The listing builds one solid part. Answer for the finished solid, in the listing's coordinates (mm). A direction names the side the tool comes from. Round coordinates to 2 decimals unless told otherwise and drop trailing zeros. Order: outer loops, then holes, each group sorted by start corner. A loop starts at its lowest first (then second) coordinate and runs counter-clockwise, first axis right, second up. Notation, with made-up numbers: (-5, 2.5) - (50, 2.5) arc R28 ccw to (50, 34.5) - close; hole circle Ø2 at (26.5, 81.25). An arc over 180 degrees is marked (long way). Write item = value, one per line.
from build123d import *

# Parameters (mm, degrees)
MODEL_W             = 85.14935
MODEL_H             = 104.19946
MODEL_W_2           = 77.14935
MODEL_H_2           = 96.19946
EXTRUDE_2_DEPTH     = 5
SKETCH_2_W          = 3.5
SKETCH_2_H          = 6
CUT_EXTRUDE_1_DEPTH = 2
SKETCH_4_W          = 91.14935
SKETCH_4_H          = 110.19946
SKETCH_4_W_2        = 85.14935
SKETCH_4_H_2        = 104.19946
EXTRUDE_5_DEPTH     = 20
FILLET_1_R          = 2
CHAMFER_1_SIZE      = 1
FILLET_2_R          = 1
CUT_EXTRUDE_2_DEPTH = 10


with BuildPart() as part:
    # Model → 凸台-拉伸2 (new body)
    with BuildSketch(Plane.XY):
        with Locations((38.194325, 47.88337)):
            Rectangle(MODEL_W, MODEL_H)
        with Locations((38.194325, 47.88337)):
            Rectangle(MODEL_W_2, MODEL_H_2, mode=Mode.SUBTRACT)
    extrude(amount=EXTRUDE_2_DEPTH)

    # 草图2 → 切除-拉伸1 (cut)
    with BuildSketch(Plane.XY.offset(5)):
        with Locations((-2.13035, 77.88337)):
            Rectangle(SKETCH_2_W, SKETCH_2_H)
        with Locations((78.519, 77.88337)):
            Rectangle(SKETCH_2_W, SKETCH_2_H)
        with Locations((-2.13035, 47.88337)):
            Rectangle(SKETCH_2_W, SKETCH_2_H)
        with Locations((78.519, 47.88337)):
            Rectangle(SKETCH_2_W, SKETCH_2_H)
        with Locations((-2.13035, 17.88337)):
            Rectangle(SKETCH_2_W, SKETCH_2_H)
        with Locations((78.519, 17.88337)):
            Rectangle(SKETCH_2_W, SKETCH_2_H)
    extrude(amount=-CUT_EXTRUDE_1_DEPTH, mode=Mode.SUBTRACT)

    # 草图4 → 凸台-拉伸5 (add)
    with BuildSketch(Plane(origin=(0, 0, 0), x_dir=(-1, 0, 0), z_dir=(0, 0, -1))):
        with Locations((-38.194325, 47.88337)):
            Rectangle(SKETCH_4_W, SKETCH_4_H)
        with Locations((-38.194325, 47.88337)):
            Rectangle(SKETCH_4_W_2, SKETCH_4_H_2, mode=Mode.SUBTRACT)
    extrude(amount=-EXTRUDE_5_DEPTH)

    # 圆角1
    fillet_1_edges = [part.edges().sort_by_distance(p)[0] for p in [
        (83.769, 102.9831, 10),
        (-7.38035, 102.9831, 10),
        (-7.38035, -7.21636, 10),
        (83.769, -7.21636, 10),
    ]]
    fillet(fillet_1_edges, radius=FILLET_1_R)

    # 倒角1
    chamfer_1_edges = [part.edges().sort_by_distance(p)[0] for p in [
        (-7.38035, 47.88337, 20),
        (38.194325, 102.9831, 20),
        (38.194325, -7.21636, 20),
        (83.769, 47.88337, 20),
        (-6.794563562, -6.630573562, 20),
        (83.183213562, -6.630573562, 20),
        (83.183213562, 102.397313562, 20),
        (-6.794563562, 102.397313562, 20),
    ]]
    chamfer(chamfer_1_edges, length=CHAMFER_1_SIZE)

    # 圆角2
    fillet_2_edges = [part.edges().sort_by_distance(p)[0] for p in [
        (-7.38035, 47.88337, 0),
        (38.194325, 102.9831, 0),
        (83.769, 47.88337, 0),
        (38.194325, -7.21636, 0),
        (-6.794563562, -6.630573562, 0),
        (83.183213562, -6.630573562, 0),
        (83.183213562, 102.397313562, 0),
        (-6.794563562, 102.397313562, 0),
    ]]
    fillet(fillet_2_edges, radius=FILLET_2_R)

    # 草图5 → 切除-拉伸2 (cut)
    with BuildSketch(Plane(origin=(76.38865, -7.21636, 20), x_dir=(-1, 0, 0), z_dir=(0, -1, 0))):
        with BuildLine():
            Line((33.694325, 13.169990539), (42.694325, 13.169990539))
            ThreePointArc((42.694325, 13.169990539), (45.094325, 10.769990539), (42.694325, 8.369990539))
            Line((42.694325, 8.369990539), (33.694325, 8.369990539))
            ThreePointArc((33.694325, 8.369990539), (31.294325, 10.769990539), (33.694325, 13.169990539))
        make_face()
    extrude(amount=-CUT_EXTRUDE_2_DEPTH, mode=Mode.SUBTRACT)


solid = part.part
Q1. Flat-ended cylindrical pins translate along their axes: P1, Ø1.8, axis at x = -2.5, y = 49, coming from the +Z side; P2, Ø3, axis at x = -2.5, y = 77, coming from the +Z side. Find the tip coordinate at first contact, or state that the pin passes through.
Model answer:
P1 = 3
P2 = 5
Q2. Section D-D on y = 56.5 is taken. Determine the outline of the cut face in (x, z), then the cut area to 3 significant figures.
Model answer:
outline = (-7.38, 1) arc R1 ccw to (-6.38, 0) - (-0.38, 0) - (-0.38, 5) - (-4.38, 5) - (-4.38, 20) - (-6.38, 20) - (-7.38, 19) - close; (76.77, 0) - (82.77, 0) arc R1 ccw to (83.77, 1) - (83.77, 19) - (82.77, 20) - (80.77, 20) - (80.77, 5) - (76.77, 5) - close
area = 159 mm^2
Q3. Find the intervals of material crossed by line 1 (X direction, y = 46.5, z = 1.75); line 2 (X direction, y = 7, z = 14); line 3 (Y direction, x = 21, z = 1.5), in increasing order. Write a range as from..to.
Model answer:
line_1 = -7.38..-0.38, 76.77..83.77
line_2 = -7.38..-4.38, 80.77..83.77
line_3 = -7.22..-0.22, 95.98..102.98
Q4. Section C-C on z = 16.5 is taken. Determine the outline of the cut face in (x, y).
Model answer:
outline = (-7.38, -5.22) arc R2 ccw to (-5.38, -7.22) - (81.77, -7.22) arc R2 ccw to (83.77, -5.22) - (83.77, 100.98) arc R2 ccw to (81.77, 102.98) - (-5.38, 102.98) arc R2 ccw to (-7.38, 100.98) - close; hole (-4.38, -4.22) - (80.77, -4.22) - (80.77, 99.98) - (-4.38, 99.98) - close
Q5. Section A-A on y = 17.5 is taken. Determine the outline of the cut face in (x, z), then the cut area to 3 significant figures.
Model answer:
outline = (-7.38, 1) arc R1 ccw to (-6.38, 0) - (-0.38, 0) - (-0.38, 3) - (-3.88, 3) - (-3.88, 5) - (-4.38, 5) - (-4.38, 20) - (-6.38, 20) - (-7.38, 19) - close; (76.77, 0) - (82.77, 0) arc R1 ccw to (83.77, 1) - (83.77, 19) - (82.77, 20) - (80.77, 20) - (80.77, 5) - (80.27, 5) - (80.27, 3) - (76.77, 3) - close
area = 145 mm^2
Q6. Determine the mould class of faces 1 (the face through (-4.38, 47, 12)), 2 (the face through (78, 78, 3)), 3 (the face through (38, -6, 6.83)) for opening direction Z: released by +Z, released by -Z, zero draft, split by the parting line, or undercut.
Model answer:
face_1 = zero draft
face_2 = released by +Z
face_3 = undercut
Q7. For faces 4 (the face through (31.295, -5.737, 9.177)), 5 (the face through (39, 102.983, 10)), 6 (the face through (-2, 78, 3)), 7 (the face through (38, 95.983, 2)), determine the directions among +Z, -Z, +X, -X, +Y, -Y from which every point of the face is accessible in a straight line to the end or side of a thin tool.
Model answer:
face_4 = -Y
face_5 = +Z, -Z, +X, -X, +Y
face_6 = +Z
face_7 = +Z, -Z
Q8. Section B-B on x = 65 is taken. Determine the outline of the cut face in (y, z), then the cut area to 3 significant figures.
Model answer:
outline = (-7.22, 1) arc R1 ccw to (-6.22, 0) - (-0.22, 0) - (-0.22, 5) - (-4.22, 5) - (-4.22, 20) - (-6.22, 20) - (-7.22, 19) - close; (95.98, 0) - (101.98, 0) arc R1 ccw to (102.98, 1) - (102.98, 19) - (101.98, 20) - (99.98, 20) - (99.98, 5) - (95.98, 5) - close
area = 159 mm^2
